Part model, mm, in its own coordinate system. Face numbers are marked on the shaded views. A direction names the side the tool comes from. Round coordinates to 2 decimals unless told otherwise and drop trailing zeros. Write each loop counter-clockwise with the first axis right and the second up, starting at its lowest first coordinate (ties: lowest second). Pieces come first, ordered by that corner, then holes. Notation, with made-up numbers: M -25,76.25 L 20,76.25 A28 cw 20,99.25 Z; hole C 79,84 d10. An arc over 180 degrees is marked long. One line per question, with ' | ' between items. Start each with the question number.
1) Saw through at D-D (z = 130). List the corners of the cut face in (x, y).
2) Wall check: probe 1 along Z at (x, y) = (259.5, -49); probe 2 along X at (y, z) = (-187, 100); probe 3 along Z at (x, y) = (180.5, -105). Give the ranges that are in metal, low to high. Write a range as [from, to].
3) Drop flat-ended pins along their axis: pin 1 Ø4 at (x, y) = (207, -152.5) entering from +Z; pin 2 Ø4.5 at (y, z) = (-103.5, 195.5) entering from -X; pin 3 Ø2.5 at (y, z) = (-145, 97.5) entering from -X. Give the stop position or say it passes through.
4) Tool access for the marked faces 1 and 2: list every direction of +Z, -Z, +X, -X, +Y, -Y with a clear straight run to the whole face (end or side of a thin tool).
5) Saw through at C-C (x = 198.5). List the corners of the cut face in (y, z), plus the area to 3 significant figures.
6) Saw through at A-A (x = 47.5). List the corners of the cut face in (y, z), plus the area to 3 significant figures.
7) Saw through at B-B (y = -24). List the corners of the cut face in (x, z).
Solid Edge part; units mm, degrees
sketch "Sketch1" plane through (0, 0, 0) normal (0, -1, 0) x (1, 0, 0)
  line L0 (77.3764, 199.2749) -> (17.3764, 199.2749)
  line L1 (17.3764, 199.2749) -> (17.3764, 196.2749)
  line L2 (17.3764, 196.2749) -> (77.3764, 196.2749)
  arc A0 (77.3764, 196.2749) -> (128.9473, 155.7325) centre (83.2091, 150.6232) cw
  arc A1 (128.9473, 155.7325) -> (179.9264, 103.2749) centre (179.9264, 154.2749) ccw
  line L3 (269.9264, 103.2749) -> (179.9264, 103.2749)
  line L4 (269.9264, 106.2749) -> (269.9264, 103.2749)
  line L5 (179.9264, 106.2749) -> (269.9264, 106.2749)
  arc A2 (131.9471, 155.6831) -> (179.9264, 106.2749) centre (179.9264, 154.2749) ccw
  arc A3 (77.3764, 199.2749) -> (131.9471, 155.6831) centre (83.2091, 150.6232) cw
  dimension "D1" = 17.3764
  dimension "D2" = 77.3764
  dimension "D3" = 179.9264
  dimension "D4" = 269.9264
  dimension "D5" = 269.9264
extrude "Protrusion1" add sketch "Sketch1" along normal blind 200
fillet "Verrundung_4" radius 3 1 edges at (269.9264, -100, 106.2749)
sketch "Sketch2" plane through (143.6514, -200, 152.9362) normal (0, -1, 0) x (1, 0, 0)
  line L0 (-126.275, 37.3386) -> (-126.275, 43.3386)
  line L1 (-126.275, 43.3386) -> (-126.275, 46.3386)
  line L2 (-126.275, 46.3386) -> (-66.275, 46.3386)
  line L3 (-66.275, 46.3386) -> (-50.0814, 44.2327)
  line L4 (-50.0814, 44.2327) -> (-37.0073, 38.973)
  line L5 (-37.0073, 38.973) -> (-35.5454, 37.3386)
  line L6 (-35.5454, 37.3386) -> (-126.275, 37.3386)
extrude "Protrusion2" add sketch "Sketch2" against normal up to vertex (200 mm away)
sketch "Sketch3" plane through (47.3764, -100, 199.2749) normal (0, 0, 1) x (1, 0, 0)
  circle A0 centre (-11.69, 90) radius 2.25
  circle A1 centre (-11.69, -90) radius 2.25
  dimension "D1" = 11.69
  dimension "D2" = 11.69
  dimension "D3" = 11.69
extrude "Cutout1" cut sketch "Sketch3" against normal through all
sketch "Sketch4" plane through (143.6514, -200, 151.449) normal (0, -1, 0) x (1, 0, 0)
  line L0 (-126.275, 47.8258) -> (-66.275, 47.8258)
  line L1 (-66.275, 47.8258) -> (-66.275, 41.8258)
  line L2 (-66.275, 41.8258) -> (-126.275, 41.8258)
  line L3 (-126.275, 41.8258) -> (-126.275, 47.8258)
extrude "Cutout2" cut sketch "Sketch4" against normal through all
sketch "Sketch5" plane through (224.9264, -100, 103.2749) normal (0, 0, -1) x (1, 0, 0)
  line L0 (-14, 100) -> (35, 100)
  line L1 (35, 100) -> (35, -80)
  line L2 (35, -80) -> (-14, -80)
  line L3 (-14, -80) -> (-14, 100)
  dimension "D1" = 14
extrude "Extrusionsausprägung_3" add sketch "Sketch5" along normal blind 8
sketch "Sketch6" plane through (47.3764, -100, 193.2749) normal (0, 0, 1) x (1, 0, 0)
  line L0 (-30, 80) -> (30, 80)
  line L1 (30, 80) -> (30, -80)
  line L2 (30, -80) -> (-30, -80)
  line L3 (-30, -80) -> (-30, 80)
  dimension "D1" = 30
extrude "Cutout3" cut sketch "Sketch6" against normal through all
sketch "Sketch7" plane through (223.4264, -100, 106.2749) normal (0, 0, 1) x (1, 0, 0)
  circle A0 centre (15.75, 62.02) radius 1.875
  circle A1 centre (15.75, -87.98) radius 1.875
  dimension "D1" = 15.75
extrude "Cutout4" cut sketch "Sketch7" against normal through all
sketch "Sketch8" plane through (224.9264, -100, 103.2749) normal (0, 0, -1) x (1, 0, 0)
  line L0 (35, 100) -> (45, 100)
  line L1 (45, 100) -> (45, -100)
  line L2 (45, -100) -> (35, -100)
  line L3 (35, -100) -> (35, 100)
extrude "Extrusionsausprägung_4" add sketch "Sketch8" along normal blind 7
sketch "Sketch9" plane through (77.3764, -100, 194.7749) normal (-1, 0, 0) x (0, -1, 0)
  line L0 (-100, 4.5) -> (-100, -1.5)
  line L1 (-100, -1.5) -> (-80, -1.5)
  line L2 (-80, -1.5) -> (-80, -4.5)
  line L3 (-80, -4.5) -> (80, -4.5)
  line L4 (80, -4.5) -> (80, -1.5)
  line L5 (80, -1.5) -> (100, -1.5)
  line L6 (100, -1.5) -> (100, 4.5)
  line L7 (100, 4.5) -> (-100, 4.5)
extrude "Extrusionsausprägung_5" add sketch "Sketch9" along normal blind 1.49
sketch "Sketch10" plane through (223.4264, -100, 106.2749) normal (0, 0, 1) x (1, 0, 0)
  line L0 (-3.5, 30) -> (6.5, 30)
  line L1 (6.5, 30) -> (6.5, -5)
  line L2 (6.5, -5) -> (11.5, -5)
  line L3 (11.5, -5) -> (1.5, -16.1803)
  line L4 (1.5, -16.1803) -> (-8.5, -5)
  line L5 (-8.5, -5) -> (-3.5, -5)
  line L6 (-3.5, -5) -> (-3.5, 30)
  dimension "D1" = 3.5
  dimension "D2" = 6.5
  dimension "D3" = 6.5
  dimension "D4" = 11.5
  dimension "D5" = 1.5
extrude "Extrusionsausschnitt_7" cut sketch "Sketch10" against normal blind 2
chamfer "Fase_1" distance 0.5 angle 60 4 edges at (33.4364, -10, 193.2749) (33.4364, -190, 193.2749) (237.3014, -37.98, 106.2749) (237.3014, -187.98, 106.2749) measured on face at (66.7198, -183.5333, 193.2748) measured on face at (66.7198, -3.5333, 193.2748) measured on face at (66.7198, -183.5333, 193.2748) measured on face at (66.7198, -3.5333, 193.2748) measured on face at (193.5564, -164.6667, 106.2749)
properties material "Nylon, allgemein"
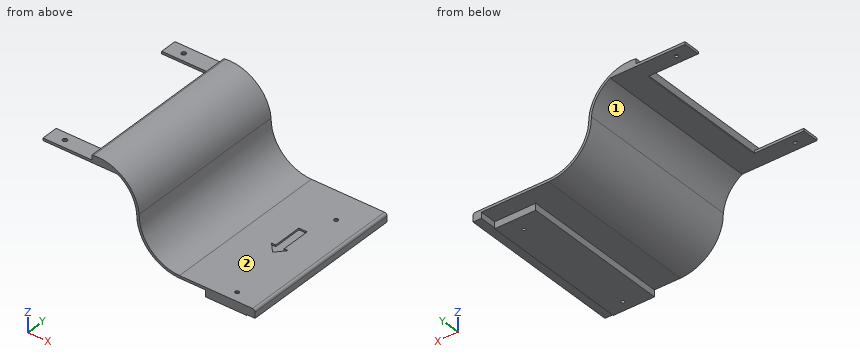
Answer key:
1) outline: M 135.07,-200 L 138.52,-200 L 138.52,0 L 135.07,0 Z
2) probe 1: z = [95.27, 106.27] | probe 2: x = [210.93, 237.58], [240.77, 269.93] | probe 3: z = [103.27, 106.27]
3) pin 1: stops at z = 106.27 | pin 2: stops at x = 75.89 | pin 3: stops at x = 210.93
4) face 1: -Z, -X, +Y, -Y | face 2: +Z, +X, +Y, -Y
5) outline: M -200,103.27 L 0,103.27 L 0,106.27 L -200,106.27 Z | area: 600 mm2
6) outline: M -200,190.27 L -180,190.27 L -180,193.27 L -200,193.27 Z; M -20,190.27 L 0,190.27 L 0,193.27 L -20,193.27 Z | area: 120 mm2
7) outline: M 75.89,190.27 L 106.57,190.27 A46.02 cw 128.95,155.73 A51 ccw 179.93,103.27 L 210.93,103.27 L 210.93,95.27 L 259.93,95.27 L 259.93,96.27 L 269.93,96.27 L 269.93,103.28 A3 ccw 266.93,106.27 L 179.93,106.27 A48 cw 131.95,155.68 A49 ccw 77.38,199.27 L 75.89,199.27 Z
